```python
from build123d import *

# Parameters (mm, degrees)
SKETCH077_W         = 42
SKETCH077_H         = 37.25
PAD024_DEPTH        = 24
SKETCH078_R         = 11
POCKET026_DEPTH     = 2
SKETCH079_W         = 134.803292
SKETCH079_H         = 4
PAD025_DEPTH        = 20
HOLE026_D           = 5
HOLE026_DEPTH       = 23.497848
HOLE026_CBORE_D     = 9
HOLE026_CBORE_DEPTH = 2
HOLE026_TIPS_R      = 2.5
HOLE027_D           = 5
HOLE027_DEPTH       = 23.497848
HOLE027_CBORE_D     = 9
HOLE027_CBORE_DEPTH = 2
HOLE027_TIPS_R      = 2.5
CHAMFER001_SIZE     = 20
SKETCH083_R         = 1.5
SKETCH083_R_2       = 6
POCKET027_DEPTH     = 5
FILLET003_R         = 1.5
FILLET004_R         = 10
FILLET005_R         = 10


with BuildPart() as part:
    # Sketch077 → Pad024 (new body)
    with BuildSketch(Plane.XY):
        Polygon((-67.401646, 0), (67.401646, 0), (67.401646, 4), (50, 4), (50, 45.25), (-50, 45.25), (-50, 4), (-67.401646, 4), align=None)
        with Locations((25, 22.625)):
            Rectangle(SKETCH077_W, SKETCH077_H, mode=Mode.SUBTRACT)
        with Locations((-25, 22.625)):
            Rectangle(SKETCH077_W, SKETCH077_H, mode=Mode.SUBTRACT)
    extrude(amount=PAD024_DEPTH)

    # Sketch078 (on Face13 of Pad024) → Pocket026 (cut)
    with BuildSketch(Plane.XZ.offset(-41.25)):
        with Locations((-25, 21)):
            Circle(SKETCH078_R)
        with Locations((25, 21)):
            Circle(SKETCH078_R)
    extrude(amount=-POCKET026_DEPTH, mode=Mode.SUBTRACT)

    # Sketch079 → Pad025 (join)
    with BuildSketch(Plane.XZ):
        with Locations((0, 22)):
            Rectangle(SKETCH079_W, SKETCH079_H)
    extrude(amount=PAD025_DEPTH)

    # Hole026
    with Locations(Plane(origin=(0, 4, 0), x_dir=(-1, 0, 0), z_dir=(0, 1, 0))):
        with Locations((58.700823, 10), (-58.700823, 10)):
            CounterBoreHole(HOLE026_D / 2, HOLE026_CBORE_D / 2, HOLE026_CBORE_DEPTH, depth=HOLE026_DEPTH)

    # Hole026 tips → Hole026 tip 1 section 0
    with BuildSketch(Plane(origin=(0, -19.497848, 0), x_dir=(-1, 0, 0), z_dir=(0, 1, 0)), mode=Mode.PRIVATE) as hole026_tip_1_s0:
        with Locations((58.700823, 10)):
            Circle(HOLE026_TIPS_R)
    loft([hole026_tip_1_s0.sketch, Vertex(-58.700823, -21, 10)], mode=Mode.SUBTRACT)

    # Hole026 tips → Hole026 tip 2 section 0
    with BuildSketch(Plane(origin=(0, -19.497848, 0), x_dir=(-1, 0, 0), z_dir=(0, 1, 0)), mode=Mode.PRIVATE) as hole026_tip_2_s0:
        with Locations((-58.700823, 10)):
            Circle(HOLE026_TIPS_R)
    loft([hole026_tip_2_s0.sketch, Vertex(58.700823, -21, 10)], mode=Mode.SUBTRACT)

    # Hole027
    with Locations(Plane.XY.offset(24)):
        with Locations((-25, -10), (25, -10)):
            CounterBoreHole(HOLE027_D / 2, HOLE027_CBORE_D / 2, HOLE027_CBORE_DEPTH, depth=HOLE027_DEPTH)

    # Hole027 tips → Hole027 tip 1 section 0
    with BuildSketch(Plane.XY.offset(0.502152), mode=Mode.PRIVATE) as hole027_tip_1_s0:
        with Locations((-25, -10)):
            Circle(HOLE027_TIPS_R)
    loft([hole027_tip_1_s0.sketch, Vertex(-25, -10, -1)], mode=Mode.SUBTRACT)

    # Hole027 tips → Hole027 tip 2 section 0
    with BuildSketch(Plane.XY.offset(0.502152), mode=Mode.PRIVATE) as hole027_tip_2_s0:
        with Locations((25, -10)):
            Circle(HOLE027_TIPS_R)
    loft([hole027_tip_2_s0.sketch, Vertex(25, -10, -1)], mode=Mode.SUBTRACT)

    # Chamfer001
    chamfer001_edges = [part.edges().sort_by_distance(p)[0] for p in [
        (-67.401646, -20, 22),
        (67.401646, -20, 22),
    ]]
    chamfer(chamfer001_edges, length=CHAMFER001_SIZE)

    # Sketch083 (on Face12 of Chamfer001) → Pocket027 (cut)
    with BuildSketch(Plane(origin=(0, 45.25, 0), x_dir=(-1, 0, 0), z_dir=(0, 1, 0))):
        with Locations((-43.253433, 4.5)):
            Circle(SKETCH083_R)
        with Locations((-12.253433, 4.5)):
            Circle(SKETCH083_R)
        with Locations((9.5, 4.5)):
            Circle(SKETCH083_R)
        with Locations((40.5, 4.5)):
            Circle(SKETCH083_R)
        with Locations((-25, 21)):
            Circle(SKETCH083_R_2)
        with Locations((25, 21)):
            Circle(SKETCH083_R_2)
    extrude(amount=-POCKET027_DEPTH, mode=Mode.SUBTRACT)

    # Fillet003
    fillet003_edges = [part.edges().sort_by_distance(p)[0] for p in [
        (0, 0, 20),
    ]]
    fillet(fillet003_edges, radius=FILLET003_R)

    # Fillet004
    fillet004_edges = [part.edges().sort_by_distance(p)[0] for p in [
        (-67.401646, 2, 0),
        (67.401646, 2, 0),
    ]]
    fillet(fillet004_edges, radius=FILLET004_R)

    # Fillet005
    fillet005_edges = [part.edges().sort_by_distance(p)[0] for p in [
        (-47.401646, -20, 22),
        (47.401646, -20, 22),
    ]]
    fillet(fillet005_edges, radius=FILLET005_R)


solid = part.part
```
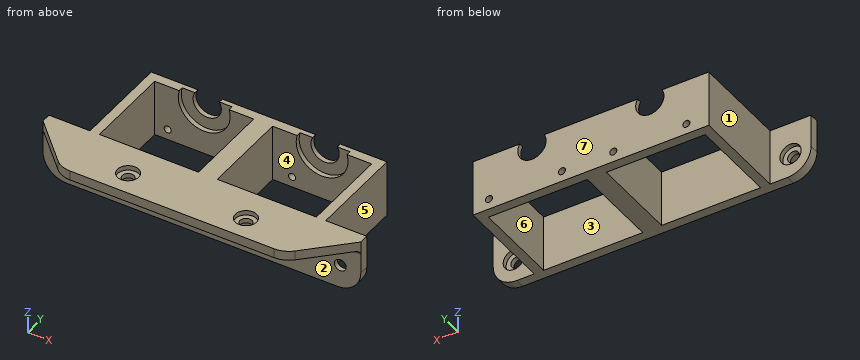
Read the model definition and answer for the solid it produces. Units are mm, in the model's axes. Face numbers are marked on the shaded views. A direction names the side the tool comes from. Coordinates: 2 decimals unless noted, no trailing zeros. Write each loop counter-clockwise with the first axis right and the second up, starting at its lowest first coordinate (ties: lowest second). Pieces come first, ordered by that corner, then holes. Notation, with made-up numbers: (40, 57.5) -> (58, 57.5) arc R20 cw to (58, 81.5) -> close; hole circle Ø3 at (3, 48). An arc over 180 degrees is marked (long way). Write item = value, one per line.
(1) Section B-B on x = -6 is taken. Write down the section's boundary in (y, z).
From the geometry:
outline = (-20, 20) -> (-1.5, 20) arc R1.5 cw to (0, 18.5) -> (0, 0) -> (4, 0) -> (4, 24) -> (-20, 24) -> close; (41.25, 0) -> (45.25, 0) -> (45.25, 24) -> (41.25, 24) -> close
(2) Straight lines are drawn through the part: L1, parallel to X at y = 19, z = 8; L2, parallel to Y at x = -11, z = 18; L3, parallel to Y at x = -25, z = 21.4. For each, find the intervals that lie inside material, in ascending order. Write a range as from..to.
From the geometry:
L1 = -50..-46, -4..4, 46..50
L2 = 0..4, 41.25..45.25
L3 = -20..-12.5, -7.5..4
(3) Section D-D on y = -10 is taken. Write down the section's boundary in (x, z), plus the area to 3 significant figures.
From the geometry:
outline = (-57.4, 20) -> (-27.5, 20) -> (-27.5, 22) -> (-29.5, 22) -> (-29.5, 24) -> (-57.4, 24) -> close; (-22.5, 20) -> (22.5, 20) -> (22.5, 22) -> (20.5, 22) -> (20.5, 24) -> (-20.5, 24) -> (-20.5, 22) -> (-22.5, 22) -> close; (27.5, 20) -> (57.4, 20) -> (57.4, 24) -> (29.5, 24) -> (29.5, 22) -> (27.5, 22) -> close
area = 403 mm2
(4) Section C-C on x = -40.5 is taken. Write down the section's boundary in (y, z), plus the area to 3 significant figures.
From the geometry:
outline = (-20, 20) -> (-1.5, 20) arc R1.5 cw to (0, 18.5) -> (0, 0) -> (4, 0) -> (4, 24) -> (-20, 24) -> close; (41.25, 0) -> (45.25, 0) -> (45.25, 3) -> (41.25, 3) -> close; (41.25, 6) -> (45.25, 6) -> (45.25, 24) -> (41.25, 24) -> close
area = 260 mm2
(5) Which of the six approach directions +Z, -Z, +X, -X, +Y, -Y give full straight-line access (tool end or side, diameter ignored) to the marked faces 1, 2 and 3?
From the geometry:
face_1 = +Z, -Z, -X, +Y
face_2 = -Z, +X, -X, -Y
face_3 = +Z, -Z
(6) Section A-A on y = 38.5 is taken. Write down the section's boundary in (x, z), plus the area to 3 significant figures.
From the geometry:
outline = (-50, 0) -> (-46, 0) -> (-46, 24) -> (-50, 24) -> close; (-4, 0) -> (4, 0) -> (4, 24) -> (-4, 24) -> close; (46, 0) -> (50, 0) -> (50, 24) -> (46, 24) -> close
area = 384 mm2
(7) For a pull along Y with two mould halves and no side action, classify the marked faces 4, 5, 6 and 7 as +Y half, -Y half, draft (parallel to the pull), parting line (faces both ways), or undercut.
From the geometry:
face_4 = undercut
face_5 = draft
face_6 = undercut
face_7 = +Y half
(8) Given pin 1 Ø6 at (y, z) = (-9.5, 20.5) entering from -X; pin 2 Ø12 at (x, z) = (18.5, 8) entering from -Y; pin 3 Ø14 at (x, z) = (58.5, 17) entering from +Y, each flat-ended and moving along its own axis, determine where each tip first touches the part or whether it passes through.
From the geometry:
pin_1 = -60.9
pin_2 = 0
pin_3 = 4
